Verification items for the finished model (mm, model axes). A direction names the side the tool comes from. Coordinates: 2 decimals unless noted, no trailing zeros. Order: outer loops, then holes, each group sorted by start corner. A loop starts at its lowest first (then second) coordinate and runs counter-clockwise, first axis right, second up. Notation, with made-up numbers: (-16, 38) -> (16, 38) arc R18 ccw to (16, 55) -> close; hole circle Ø9 at (-20.5, -12.5). An arc over 180 degrees is marked (long way). Answer as CSV lines item,"result".
Autodesk Fusion 360 part; units mm, degrees
sketch "Sketch1" plane through (0, 0, 0) normal (1, 0, 0) x (0, 0, -1)
  line L0 (-50, 30) -> (50, 30)
  line L1 (50, 30) -> (50, -30)
  line L2 (50, -30) -> (-50, -30)
  line L3 (-50, -30) -> (-50, 30)
  line L4 (48, -28) -> (-48, -28)
  line L5 (-48, -28) -> (-48, 28)
  line L6 (-48, 28) -> (48, 28)
  line L7 (48, 28) -> (48, -28)
  dimension "d1" = 100
  dimension "d2" = 60
  dimension "d3" = 2
  dimension "d17" = 30
  dimension "d18" = 50
extrude "Extrude1" add sketch "Sketch1" along normal blind 2 contours L0 L1 L2 L3 | L4 L5 L6 L7
extrude "Extrude2" add sketch "Sketch1" against normal blind 15
sketch "Sketch2" plane through (0, 0, 0) normal (-1, 0, 0) x (0, 0, 1)
  line L0 (-48, 28) -> (-48, -28)
  line L1 (-48, -28) -> (48, -28)
  line L2 (48, -28) -> (48, 28)
  line L3 (48, 28) -> (-48, 28)
  line L4 (45, 25) -> (-45, 25)
  line L5 (-45, 25) -> (-45, -25)
  line L6 (-45, -25) -> (45, -25)
  line L7 (45, -25) -> (45, 25)
  line L8 (45, 25) -> (-45, -25) construction
  line L9 (-45, 25) -> (45, -25) construction
  dimension "d8" = 90
  dimension "d9" = 50
extrude "Extrude3" add sketch "Sketch2" along normal blind 13 contours L4 L5 L6 L7
sketch "Sketch4" plane through (2, 0, 0) normal (1, 0, 0) x (0, 0, -1)
  line L0 (-50, -30) -> (50, -30)
  line L1 (50, -30) -> (50, 30)
  line L2 (50, 30) -> (-50, 30)
  line L3 (-50, 30) -> (-50, -30)
  line L4 (-50, 10) -> (150, 10)
  line L5 (150, 10) -> (150, -10)
  line L6 (150, -10) -> (-50, -10)
  line L7 (-50, -10) -> (-50, 10)
extrude "Extrude4" add sketch "Sketch4" along normal blind 6 contours L1 L3 L4 L6 L7 | L1 L4 L5 L6
sketch "Sketch5" plane through (0, -10, 0) normal (0, -1, 0) x (1, 0, 0)
  line L0 (2, -50) -> (2, -150)
  line L1 (2, -150) -> (8, -150)
  line L2 (8, -150) -> (8, 50)
  line L3 (8, 50) -> (2, 50)
  line L4 (2, 50) -> (2, -50)
  line L5 (28, -115) -> (28, -85)
  line L6 (28, -85) -> (8, -85)
  arc A0 (8, -115) -> (28, -115) centre (18, -115) ccw
  circle A1 centre (18, -115) radius 3
  dimension "d28" = 6
extrude "Extrude5" add sketch "Sketch5" against normal blind 10 from surface at -5 contours L2 L5 L6 A0
Item 1: Section check C-C, the plane x = 18. Record the boundary of the cut face in (y, z).
Answer list:
outline,"(-5, -125) -> (5, -125) -> (5, -118) -> (-5, -118) -> close; (-5, -112) -> (5, -112) -> (5, -85) -> (-5, -85) -> close"
Item 2: Section check D-D, the plane z = 15. Record the boundary of the cut face in (x, y).
Answer list:
outline,"(-15, -30) -> (2, -30) -> (2, -10) -> (8, -10) -> (8, 10) -> (2, 10) -> (2, 30) -> (-15, 30) -> (-15, 28) -> (0, 28) -> (0, 25) -> (-13, 25) -> (-13, -25) -> (0, -25) -> (0, -28) -> (-15, -28) -> close"
Item 3: Section check B-B, the plane y = 2. Record the boundary of the cut face in (x, z).
Answer list:
outline,"(-15, -50) -> (2, -50) -> (2, -150) -> (8, -150) -> (8, -115) arc R10 ccw to (28, -115) -> (28, -85) -> (8, -85) -> (8, 50) -> (-15, 50) -> (-15, 48) -> (0, 48) -> (0, 45) -> (-13, 45) -> (-13, -45) -> (0, -45) -> (0, -48) -> (-15, -48) -> close; hole circle Ø6 at (18, -115)"
Item 4: Depth check by flat-ended pin: pin 1 Ø2 at (x, z) = (4, 13) entering from +Y; pin 2 Ø11 at (x, y) = (16.5, 2) entering from +Z; pin 3 Ø16.5 at (x, y) = (-8.5, -9.5) entering from -Z. Enter the tip coordinate at first touch or a pass-through.
Answer list:
pin 1,"y = 10"
pin 2,"z = -85"
pin 3,"z = -50"
Item 5: Release check for a two-part mould opening along Z. For faces 1 (the flat face through (5, 10, -49)), 2 (the flat face through (-6, 0, 50)), 3 (the flat face through (-7, 0, 48)) record: +Z half, -Z half, draft (parallel to the pull), parting line (faces both ways), or undercut.
Answer list:
face 1,"draft"
face 2,"+Z half"
face 3,"undercut"
Item 6: Section check A-A, the plane x = -10.5. Record the boundary of the cut face in (y, z).
Answer list:
outline,"(-30, -50) -> (30, -50) -> (30, 50) -> (-30, 50) -> close; (-25, -45) -> (25, -45) -> (25, 45) -> (-25, 45) -> close; hole (-28, -48) -> (28, -48) -> (28, 48) -> (-28, 48) -> close"
Item 7: Thickness scan on line 1 (Z direction, x = -11, y = 17.5); line 2 (Y direction, x = -11, z = -31); line 3 (Z direction, x = 18, y = 2). Record the ranges inside material, lowest first.
Answer list:
line 1,"-50 to -48, -45 to 45, 48 to 50"
line 2,"-30 to -28, -25 to 25, 28 to 30"
line 3,"-125 to -118, -112 to -85"
Item 8: Tool access check on faces 4 (the flat face through (-7, -28, -1)), 5 (the flat face through (5, -10, -51)), 6 (the flat face through (2, 20, 1)). Record the directions out of +Z, -Z, +X, -X, +Y, -Y that give a thin tool (end or side, any length) a straight path to the whole face; none if there is none.
Answer list:
face 4,"-X"
face 5,"+Z, -Z, +X, -Y"
face 6,"+Z, -Z, +X, +Y"
